Source: CAD feature listing. Evaluate the final solid. Frame: model axes, mm. Face numbers are marked on the shaded views. Round coordinates to 2 decimals unless told otherwise and drop trailing zeros. Loops run counter-clockwise (first coordinate to the right, second up) from the corner with the lowest first, then second, coordinate; pieces in that order, holes last. Notation, with made-up numbers: M 19,-15.75 L 32,-15.75 A7 ccw 32,-3.75 Z; hole C 1.5,68 d7. An arc over 180 degrees is marked long. Write each question's results on one line, items separated by ' | '. Start each with the question number.
1. Section B-B on x = 0. Output: boundary loops of the cut face in (y, z).
2. Contact query for flat-ended pins moving along their axis: pin 1 Ø4 at (y, z) = (-3.5, 4) entering from +X; pin 2 Ø8 at (y, z) = (-2, -8) entering from +X; pin 3 Ø10 at (y, z) = (-27, -9) entering from -X; pin 4 Ø6 at (x, z) = (-19.5, 27.5) entering from +Y. Output: stop coordinate, or through.
3. Section D-D on z = 28.5. Output: boundary loops of the cut face in (x, y), and give its area (3 significant figures).
4. Draft query along Z for the marked faces 1 and 2. Return one class per face: released by +Z, released by -Z, zero draft, split by the parting line, or undercut.
5. Ray query, line 1 (X direction, y = 8, z = 0); line 2 (Y direction, x = -36.75, z = 0); line 3 (Z direction, x = -0.5, y = -23.5). Return the intervals inside material, ascending.
6. Section C-C on y = 0. Output: boundary loops of the cut face in (x, z).
7. Section A-A on z = 0. Output: boundary loops of the cut face in (x, y), and give its area (3 significant figures).
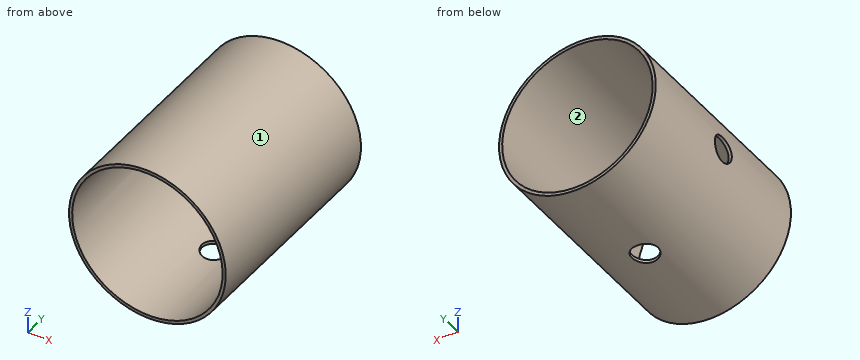
from build123d import *

# Parameters (mm, degrees)
SKETCH1_R           = 38.1
SKETCH1_R_2         = 36.576
BOSS_EXTRUDE1_DEPTH = 50.8
SKETCH2_R           = 6.35
CUT_EXTRUDE1_DEPTH  = 75.053089065
SKETCH3_R           = 6.35
CUT_EXTRUDE2_DEPTH  = 75.053089236


with BuildPart() as part:
    # Sketch1 → Boss-Extrude1 (new, symmetric)
    with BuildSketch(Plane(origin=(0, 0, 0), x_dir=(1, 0, 0), z_dir=(0, 1, 0))):
        with Locations(Location((0, 0, 0), (0, 0, 270))):
            Circle(SKETCH1_R)
        with Locations(Location((0, 0, 0), (0, 0, 270))):
            Circle(SKETCH1_R_2, mode=Mode.SUBTRACT)
    extrude(amount=BOSS_EXTRUDE1_DEPTH, both=True)

    # Sketch2 → Cut-Extrude1 (cut, through all)
    with BuildSketch(Plane(origin=(0, 0, 0), x_dir=(0, 0, -1), z_dir=(1, 0, 0))):
        Circle(SKETCH2_R)
    extrude(amount=-CUT_EXTRUDE1_DEPTH, mode=Mode.SUBTRACT)

    # Sketch3 → Cut-Extrude2 (cut, through all)
    with BuildSketch(Plane.XY):
        with Locations(Location((0, 0, 0), (0, 0, 90))):
            Circle(SKETCH3_R)
    extrude(amount=-CUT_EXTRUDE2_DEPTH, mode=Mode.SUBTRACT)


solid = part.part
Taken from the geometry:
1) outline: M -50.8,-38.1 L -6.35,-38.1 L -6.35,-36.58 L -50.8,-36.58 Z; M -50.8,36.58 L 50.8,36.58 L 50.8,38.1 L -50.8,38.1 Z; M 6.35,-38.1 L 50.8,-38.1 L 50.8,-36.58 L 6.35,-36.58 Z
2) pin 1: x = 38.05 | pin 2: x = 37.89 | pin 3: x = -37.89 | pin 4: y = 50.8
3) outline: M -25.29,-50.8 L -22.92,-50.8 L -22.92,50.8 L -25.29,50.8 Z; M 22.92,-50.8 L 25.29,-50.8 L 25.29,50.8 L 22.92,50.8 Z | area: 480 mm^2
4) face 1: split by the parting line | face 2: undercut
5) line 1: -38.1 to -36.58, 36.58 to 38.1 | line 2: -50.8 to -6.35, 6.35 to 50.8 | line 3: -38.1 to -36.57, 36.57 to 38.1
6) outline: M -37.57,-6.35 A38.1 ccw -6.35,-37.57 L -6.35,-36.02 A36.58 cw -36.02,-6.35 Z; M -37.57,6.35 L -36.02,6.35 A36.58 cw long 6.35,-36.02 L 6.35,-37.57 A38.1 ccw long Z
7) outline: M -38.1,-50.8 L -36.58,-50.8 L -36.58,-6.35 L -38.1,-6.35 Z; M -38.1,6.35 L -36.58,6.35 L -36.58,50.8 L -38.1,50.8 Z; M 36.58,-50.8 L 38.1,-50.8 L 38.1,50.8 L 36.58,50.8 Z | area: 290 mm^2
